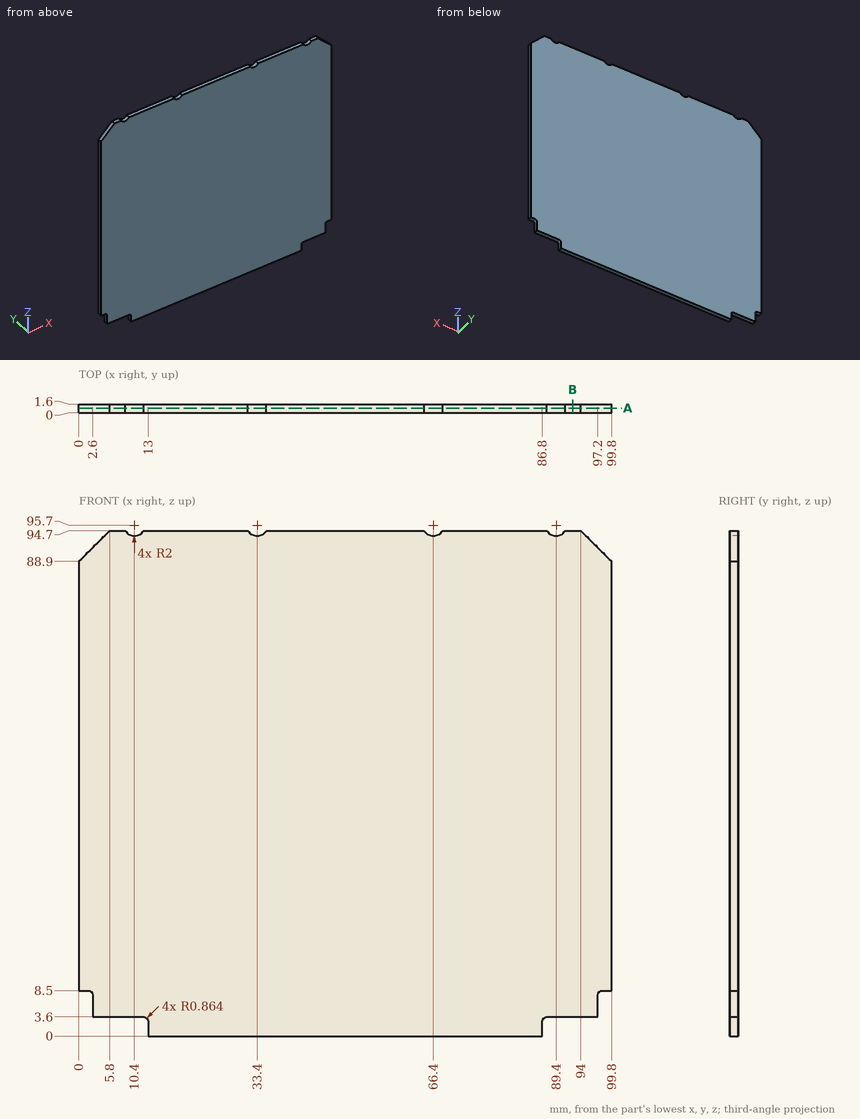
For this review, use the dimensioned drawing (mm, ordinates from the lowest corner) and the shaded views. Give positions to 0.01 mm unless a question says otherwise; leave off trailing zeros. Order: outer loops, then holes, each group sorted by start corner. A loop starts at its lowest first (then second) coordinate and runs counter-clockwise, first axis right, second up. Notation, with made-up numbers: (39, 36.5) - (55, 36.5) arc R21 ccw to (55, 52.5) - close; hole circle Ø6 at (-0.5, -37). An arc over 180 degrees is marked (long way). Use CSV: the item, a comma, the result in double quotes. Start each with the question number.
Q1. For P1, Ø0.5, axis at y = 0.5, z = 5.5, coming from the -X side; P2, Ø0.5, axis at y = 1, z = 1, coming from the +X side; P3, Ø0.8, axis at y = 1, z = 6.5, coming from the +X side, all flat-tipped, find the tip position at first contact; note any pin that passes through.
Q2. Take a section at B-B (x = 92.5). State the section outline as (y, z) points, and give its area (3 significant figures).
Q3. Take a section at A-A (y = 0.85). State the section outline as (x, z) points.
Q4. For line 1 (Z direction, x = 7, y = 0.75); line 2 (Z direction, x = 95, y = 0.25); line 3 (X direction, y = 0.55, z = 89), list the stretches that pass through material, from the lowest coordinate up.
Calculated:
1,P1,"stops at x = 2.6"
1,P2,"stops at x = 86.8"
1,P3,"stops at x = 97.2"
2,outline,"(0, 3.6) - (1.6, 3.6) - (1.6, 94.7) - (0, 94.7) - close"
2,area,"146 mm²"
3,outline,"(0, 8.5) - (1.74, 8.5) arc R0.86 cw to (2.6, 7.64) - (2.6, 3.6) - (12.14, 3.6) arc R0.86 cw to (13, 2.74) - (13, 0) - (86.8, 0) - (86.8, 2.74) arc R0.86 cw to (87.66, 3.6) - (97.2, 3.6) - (97.2, 7.64) arc R0.86 cw to (98.06, 8.5) - (99.8, 8.5) - (99.8, 88.9) - (94, 94.7) - (91.13, 94.7) arc R2 cw to (87.67, 94.7) - (68.13, 94.7) arc R2 cw to (64.67, 94.7) - (35.13, 94.7) arc R2 cw to (31.67, 94.7) - (12.13, 94.7) arc R2 cw to (8.67, 94.7) - (5.8, 94.7) - (0, 88.9) - close"
4,line 1,"z = 3.6 to 94.7"
4,line 2,"z = 3.6 to 93.7"
4,line 3,"x = 0.1 to 99.7"
